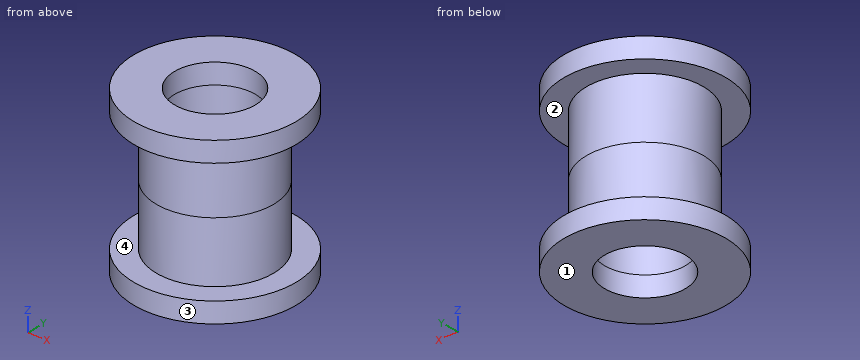
Autodesk Inventor part; units mm, degrees
ref_plane "YZ Plane" through (0, 0, 0) normal (1, 0, 0) x (0, 1, 0)
ref_plane "XZ Plane" through (0, 0, 0) normal (0, 1, 0) x (-1, 0, 0)
ref_plane "XY Plane" through (0, 0, 0) normal (0, 0, 1) x (1, 0, 0)
sketch "Sketch1" plane through (0, 0, 0) normal (0, 0, 1) x (1, 0, 0)
  line L0 (-12.7, 76.2) -> (12.7, 76.2) construction
  line L1 (12.7, 76.2) -> (12.7, -76.2) construction
  line L2 (12.7, -76.2) -> (-12.7, -76.2) construction
  line L3 (-12.7, -76.2) -> (-12.7, 76.2) construction
  line L4 (-12.7, 76.2) -> (12.7, -76.2) construction
  line L5 (12.7, 76.2) -> (-12.7, -76.2) construction
  line L6 (19.05, 76.2) -> (44.45, 76.2) construction
  line L7 (44.45, 76.2) -> (44.45, -76.2) construction
  line L8 (44.45, -76.2) -> (19.05, -76.2) construction
  line L9 (19.05, -76.2) -> (19.05, 76.2) construction
  line L10 (19.05, 76.2) -> (44.45, -76.2) construction
  line L11 (44.45, 76.2) -> (19.05, -76.2) construction
  circle A0 centre (3.8735, 0) radius 6.35
  line L12 (11.1125, -57.0186) -> (11.1125, 57.0186) construction
  line L13 (11.1125, 57.0186) -> (-14.2875, -95.3814) construction
  line L14 (-14.2875, -95.3814) -> (-14.2875, 95.3814) construction
  line L15 (-14.2875, 95.3814) -> (11.1125, -57.0186) construction
  line L16 (13.081, 27.2802) -> (13.081, -0.0011) construction
  circle A1 centre (3.8735, 0) radius 9.2075
  point P0 (0, 0)
  point P1 (31.75, 0)
  point P2 (0, 0)
  point P3 (0, 76.2)
  point P4 (31.75, 76.2)
  point P5 (0, 0)
  dimension "d1" = 25.4
  dimension "d2" = 152.4
  dimension "d3" = 25.4
  dimension "d4" = 152.4
  dimension "d5" = 6.35
  dimension "d6" = 12.7
  dimension "d7" = 1.5875
  dimension "d8" = 0.381
  dimension "d11" = 18.415
  dimension "d21" = 8.8265
extrude "Extrusion1" add sketch "Sketch1" along normal mid plane 19.05
sketch "Sketch2" plane through (3.8735, 0, 9.525) normal (0, 0, 1) x (1, 0, 0)
  circle A0 centre (0, 0) radius 9.2075
  circle A1 centre (0, 0) radius 12.7
  circle A2 centre (0, 0) radius 6.35
  point P0 (-3.8735, 0)
  dimension "d23" = 25.4
extrude "Extrusion2" add sketch "Sketch2" along normal blind 3.175 contours A0 | A1
sketch "Sketch3" plane through (3.8735, 0, -9.525) normal (0, 0, -1) x (-1, 0, 0)
  circle A0 centre (0, 0) radius 9.2075
  circle A1 centre (0, 0) radius 12.7
  circle A2 centre (0, 0) radius 6.35
  point P0 (3.8735, 0)
  dimension "d22" = 25.4
extrude "Extrusion3" add sketch "Sketch3" along normal blind 3.175 contours A0 | A1
properties part number "EL2-007" material "Aluminum 6061"
The model under review builds one solid part; all positions refer to its coordinate system, in mm. Face numbers are marked on the shaded views. Give positions to 0.01 mm unless a question says otherwise; leave off trailing zeros. Loops run counter-clockwise (first coordinate to the right, second up) from the corner with the lowest first, then second, coordinate; pieces in that order, holes last. Notation, with made-up numbers: (-23, 20.25) -> (-6, 20.25) arc R16 ccw to (-6, 40.25) -> close; hole circle Ø1 at (-14, 56). An arc over 180 degrees is marked (long way). Use CSV: the item, a comma, the result in double quotes.
1. Consider section B-B, the plane x = 2.5. Write out the cut boundary in (y, z) (1 decimal), then the cut area to 3 significant figures.
Result:
outline,"(-12.6, -12.7) -> (-6.2, -12.7) -> (-6.2, 12.7) -> (-12.6, 12.7) -> (-12.6, 9.5) -> (-9.1, 9.5) -> (-9.1, -9.5) -> (-12.6, -9.5) -> close; (6.2, -12.7) -> (12.6, -12.7) -> (12.6, -9.5) -> (9.1, -9.5) -> (9.1, 9.5) -> (12.6, 9.5) -> (12.6, 12.7) -> (6.2, 12.7) -> close"
area,"192 mm²"
2. To check wall thickness, follow probe 1 along Z at (x, y) = (14.5, -5.75) (3 decimals); probe 2 along Y at (x, z) = (4, 6.75); probe 3 along Y at (x, z) = (7.75, -6.5). State the ranges of each line that lie inside material, in increasing order. Write a range as from..to.
Result:
probe 1,"z = -12.7..-9.525, 9.525..12.7"
probe 2,"y = -9.21..-6.35, 6.35..9.21"
probe 3,"y = -8.35..-5.03, 5.03..8.35"
3. The part is to be moulded in two halves that separate along Z. For the marked faces 1, 2, 3 and 4, say which applies: +Z half, -Z half, draft (parallel to the pull), parting line (faces both ways), or undercut.
Result:
face 1,"-Z half"
face 2,"undercut"
face 3,"draft"
face 4,"undercut"
4. Consider section D-D, the plane y = 8.5. Write out the cut boundary in (x, z) (3 decimals), then the cut area to 3 significant figures.
Result:
outline,"(-5.563, -12.7) -> (13.31, -12.7) -> (13.31, -9.525) -> (7.413, -9.525) -> (7.413, 9.525) -> (13.31, 9.525) -> (13.31, 12.7) -> (-5.563, 12.7) -> (-5.563, 9.525) -> (0.334, 9.525) -> (0.334, -9.525) -> (-5.563, -9.525) -> close"
area,"255 mm²"
5. For P1, Ø1.5, axis at y = 0, z = 6.5, coming from the +X side; P2, Ø5, axis at x = 0, z = 0.5, coming from the -Y side; P3, Ø14.5, axis at x = 3.87, y = 0, coming from the -Z side; P4, Ø12, axis at y = 8.5, z = -2, coming from the +X side, all flat-tipped, find the tip position at first contact; note any pin that passes through.
Result:
P1,"stops at x = 13.08"
P2,"stops at y = -9.1"
P3,"stops at z = -12.7"
P4,"stops at x = 12.74"
6. Consider section A-A, the plane y = 0. Write out the cut boundary in (x, z) (1 decimal).
Result:
outline,"(-8.8, -12.7) -> (-2.5, -12.7) -> (-2.5, 12.7) -> (-8.8, 12.7) -> (-8.8, 9.5) -> (-5.3, 9.5) -> (-5.3, -9.5) -> (-8.8, -9.5) -> close; (10.2, -12.7) -> (16.6, -12.7) -> (16.6, -9.5) -> (13.1, -9.5) -> (13.1, 9.5) -> (16.6, 9.5) -> (16.6, 12.7) -> (10.2, 12.7) -> close"
